Autodesk Inventor part; units mm, degrees
ref_plane "YZ Plane" through (0, 0, 0) normal (1, 0, 0) x (0, 1, 0)
ref_plane "XZ Plane" through (0, 0, 0) normal (0, 1, 0) x (-1, 0, 0)
ref_plane "XY Plane" through (0, 0, 0) normal (0, 0, 1) x (1, 0, 0)
sketch "Boceto1" plane through (0, 0, 0) normal (0, 1, 0) x (-1, 0, 0)
  line L0 (0, 0) -> (70, 0)
  line L1 (70, 0) -> (70, 30)
  line L2 (70, 30) -> (0, 30)
  line L3 (0, 30) -> (0, 0)
  line L4 (0, 30) -> (10, 30)
  line L5 (10, 30) -> (10, 36)
  line L6 (10, 36) -> (0, 36)
  line L7 (0, 36) -> (0, 30)
  dimension "d0" = 10
  dimension "d14" = 70
extrude "Extrusión1" add sketch "Boceto1" along normal blind 4
sketch "Boceto2" plane through (0, 4, 0) normal (0, 1, 0) x (1, 0, 0)
  line L0 (-10, -30) -> (-6, -30)
  line L1 (-6, -30) -> (-6, -36)
  line L2 (-6, -36) -> (-10, -36)
  line L3 (-10, -36) -> (-10, -30)
extrude "Extrusión2" add sketch "Boceto2" along normal blind 4
chamfer "Chaflán1" distance 20 angle 45 1 edges at (-70, 2, 30)
sketch "Boceto6" plane through (0, 4, 0) normal (0, 1, 0) x (1, 0, 0)
  line L0 (-70, 0) -> (-50, 0)
  line L1 (-50, 0) -> (-50, -4)
  line L2 (-50, -4) -> (-70, -4)
  line L3 (-70, -4) -> (-70, 0)
  dimension "d15" = 20
extrude "Extrusión4" add sketch "Boceto6" along normal blind 30
chamfer "Chaflán2" distance 10 angle 45 1 edges at (-50, 34, 2)
sketch "Boceto7" plane through (0, 0, 0) normal (0, -1, 0) x (1, 0, 0)
  line L0 (-70, 0) -> (-50, 0)
  line L1 (-50, 0) -> (-50, 4)
  line L2 (-50, 4) -> (-70, 4)
  line L3 (-70, 4) -> (-70, 0)
  dimension "d19" = 20
extrude "Extrusión5" add sketch "Boceto7" along normal blind 30
sketch "Boceto8" plane through (0, 0, 0) normal (0, -1, 0) x (1, 0, 0)
  line L0 (-10, 36) -> (0, 36)
  line L1 (-10, 30) -> (-6, 30)
  line L2 (-6, 30) -> (-6, 36)
  line L3 (-6, 36) -> (-10, 36)
  line L4 (-10, 36) -> (-10, 30)
extrude "Extrusión6" add sketch "Boceto8" along normal blind 4
chamfer "Chaflán3" distance 10 angle 45 1 edges at (-50, -30, 2)
sketch "Boceto9" plane through (0, 0, 0) normal (0, -1, 0) x (1, 0, 0)
  line L0 (0, 36) -> (0, 0)
  line L1 (0, 0) -> (0, 4)
  line L2 (0, 4) -> (-10, 4)
  line L3 (-10, 4) -> (-10, 0)
  line L4 (-10, 0) -> (0, 0)
extrude "Extrusión7" add sketch "Boceto9" along normal blind 25
sketch "Boceto10" plane through (0, 4, 0) normal (0, 1, 0) x (1, 0, 0)
  line L0 (0, -36) -> (0, 0)
  line L1 (0, 0) -> (0, -4)
  line L2 (0, -4) -> (-10, -4)
  line L3 (-10, -4) -> (-10, 0)
  line L4 (-10, 0) -> (0, 0)
extrude "Extrusión8" add sketch "Boceto10" along normal blind 25
chamfer "Chaflán4" distance 5 angle 45 4 edges at (-60, 0, 4) (-5, 0, 4) (-60, 4, 4) (-5, 4, 4)
chamfer "Chaflán5" distance 4 angle 45 2 edges at (-8, 4, 30) (-8, 0, 30)
properties part number "Pata"
For this review, take the finished solid that the model builds, in its own axes (mm). A direction names the side the tool comes from. Give positions to 0.01 mm unless a question says otherwise; leave off trailing zeros. Write each loop counter-clockwise with the first axis right and the second up, starting at its lowest first coordinate (ties: lowest second). Pieces come first, ordered by that corner, then holes.
Item 1: Take a section at B-B (z = 8). Give the boundary of the cut face in (x, y), and give its area (3 significant figures).
Item 2: Wall thickness on probe 1 along Y at (x, z) = (-5.5, 13); probe 2 along Z at (x, y) = (-53, -1); probe 3 along Z at (x, y) = (-55, 6): over which ranges is each line inside the solid? List them lowest first.
Item 3: Machinability: for faces 1 (the face through (-60, 21, 4)), 2 (the face through (-60, -17, 4)), 3 (the face through (-5, -2, 7)), 4 (the face through (-6, -2, 32)), which of the approach directions +Z, -Z, +X, -X, +Y, -Y give a long, thin tool a straight path to every point of the face, cutting with its end or side? Answer none if there is none.
Item 4: Take a section at C-C (x = -63). Give the boundary of the cut face in (y, z), and give its area (3 significant figures).
Item 5: The part is to be moulded in two halves that separate along Z. For faces 5 (the face through (-8, 6, 28)), 6 (the face through (-5, 29, 2)), 7 (the face through (-5, 19, 4)), say which applies: +Z half, -Z half, draft (parallel to the pull), parting line (faces both ways), or undercut.
Item 6: Take a section at D-D (y = 6.5). Give the boundary of the cut face in (x, z).
Item 7: Insertion check: P1, Ø8, axis at x = -54, z = 14, coming from the -Y side; P2, Ø1.2, axis at x = -3, z = 2.5, coming from the +Y side; P3, Ø22, axis at x = -58, y = 23, coming from the +Z side. Each pin has a flat end and moves straight along its axis. Give the tip position at first contact, or say it passes through.
Item 8: Take a section at A-A (y = -16.5). Give the boundary of the cut face in (x, z), and give its area (3 significant figures).
Established:
1. outline: (-70, -1) - (-50, -1) - (-50, 0) - (-10, 0) - (-10, -1) - (0, -1) - (0, 5) - (-10, 5) - (-10, 4) - (-50, 4) - (-50, 5) - (-70, 5) - close
1. area: 340 mm2
2. probe 1: y = 0 to 4
2. probe 2: z = 0 to 8
2. probe 3: z = 0 to 7
3. face 1: +Z, +X, -X, +Y
3. face 2: +Z, +X, -X, -Y
3. face 3: +X, -X, -Y
3. face 4: +Z, +X, -Y
4. outline: (-30, 0) - (34, 0) - (34, 4) - (9, 4) - (4, 9) - (4, 17) - (0, 17) - (0, 9) - (-5, 4) - (-30, 4) - close
4. area: 333 mm2
5. face 5: undercut
5. face 6: draft
5. face 7: +Z half
6. outline: (-70, 0) - (-50, 0) - (-50, 6.5) - (-70, 6.5) - close; (-10, 0) - (0, 0) - (0, 6.5) - (-10, 6.5) - close; (-10, 28.5) - (-6, 28.5) - (-6, 36) - (-10, 36) - close
7. P1: stops at y = 0
7. P2: stops at y = 29
7. P3: stops at z = 4
8. outline: (-70, 0) - (-50, 0) - (-50, 4) - (-70, 4) - close; (-10, 0) - (0, 0) - (0, 4) - (-10, 4) - close
8. area: 120 mm2
